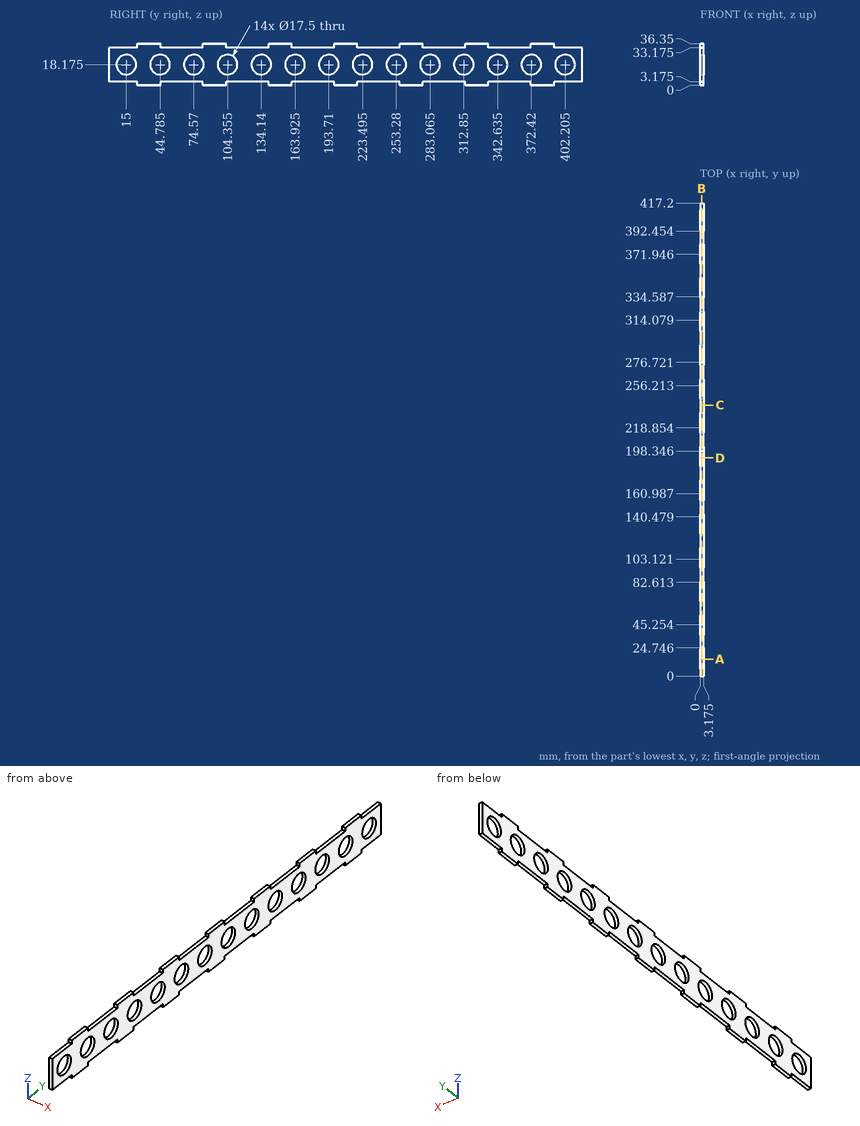
Drawing for the job (mm, zero at the part's lowest x, y, z). Round coordinates to 2 decimals unless told otherwise and drop trailing zeros. Order: outer loops, then holes, each group sorted by start corner. A loop starts at its lowest first (then second) coordinate and runs counter-clockwise, first axis right, second up. Notation, with made-up numbers: (69, -39) -> (112, -39) arc R7 ccw to (112, -29) -> close; hole circle Ø9 at (-1.5, 56.5). An arc over 180 degrees is marked (long way). Write item = value, one per line. Start each with the question number.
(1) Cut at D-D, the plane y = 192.5. List the corners of the cut face in (x, z) (1 decimal).
(2) Cut at A-A, the plane y = 15. List the corners of the cut face in (x, z) (1 decimal), then the cut area to 3 significant figures.
(3) Cut at C-C, the plane y = 239. List the corners of the cut face in (x, z) (1 decimal).
(4) Pin check, flat tips, straight feed: P1, Ø1.6, axis at x = 2, y = 245, coming from the -Z side (3 decimals); P2, Ø1.6, axis at x = 1, z = 2, coming from the +Y side. Stop position of each tip, or through.
(5) Probe line 1 (Z direction, x = 0.85, y = 134.14) (1 decimal); line 2 (Z direction, x = 0.45, y = 62.5) (1 decimal); line 3 (Z direction, x = 2.95, y = 106.5) (1 decimal). List the from-to ranges inside material, lowest first. Write a range as [from, to].
(6) Cut at B-B, the plane x = 1.35. State how many separate pieces and enclosed holes the cut face has, then the cut area to 3 significant figures.
Model answer:
q1.outline = (0, 3.2) -> (3.2, 3.2) -> (3.2, 9.5) -> (0, 9.5) -> close; (0, 26.8) -> (3.2, 26.8) -> (3.2, 33.2) -> (0, 33.2) -> close
q2.outline = (0, 3.2) -> (3.2, 3.2) -> (3.2, 9.4) -> (0, 9.4) -> close; (0, 26.9) -> (3.2, 26.9) -> (3.2, 33.2) -> (0, 33.2) -> close
q2.area = 39.7 mm2
q3.outline = (0, 3.2) -> (3.2, 3.2) -> (3.2, 33.2) -> (0, 33.2) -> close
q4.P1 = 3.175
q4.P2 = 392.45
q5.line_1 = [3.2, 9.4], [26.9, 33.2]
q5.line_2 = [3.2, 33.2]
q5.line_3 = [3.2, 9.7], [26.7, 33.2]
q6.separate_pieces = 1
q6.enclosed_holes = 14
q6.area = 10,100 mm2
